For this review, take the finished solid that the model builds, in its own axes (mm). A direction names the side the tool comes from. Coordinates: 2 decimals unless noted, no trailing zeros. Write each loop counter-clockwise with the first axis right and the second up, starting at its lowest first coordinate (ties: lowest second). Pieces come first, ordered by that corner, then holes.
1) Insertion check: P1, Ø3, axis at x = 1.5, z = 10.5, coming from the -Y side; P2, Ø1.2, axis at y = 0, z = 13.5, coming from the +X side; P3, Ø1, axis at x = 1.5, z = 12.5, coming from the +Y side; P4, Ø1.6, axis at x = 0, y = 0, coming from the -Z side. Each pin has a flat end and moves straight along its axis. Give the tip position at first contact, or say it passes through.
2) Mouldability with a two-part tool opening along X and no side actions: class faces 4 (the face through (-3.45, 0, 8)), 5 (the face through (-1.3, 1.3, 0)), 6 (the face through (0, 0, 9)) as pulls with the +X half, pulls with the -X half, needs draft (parallel to the pull), parting line crosses it, or undercut.
3) We need section B-B on z = 6.25. Write out the cut boundary in (x, y).
4) We need section C-C on z = 13.5. Write out the cut boundary in (x, y), then the cut area to 3 significant figures.
5) To check wall thickness, follow line 1 along Z through (x, y) = (0.95, 0); line 2 along Z through (x, y) = (-1, -2.75); line 3 along Y through (x, z) = (0, 3.5). State the ranges of each line that lie inside material, in increasing order.
6) For faces 1 (the face through (1.7, 3, 7.7)), 2 (the face through (-0.17, -1.29, 4.7)), 3 (the face through (-2, -2, 10)), list the 3-axis set-ups (+Z, -Z, +X, -X, +Y, -Y) from which the entire face can be reached by the end or side of a thin tool; tool diameter is ignored.
from build123d import *

# Parameters (mm, degrees)
F2_R          = 5.941705
F3_DEPTH      = 16.501
F4_R          = 0.75
F5_DEPTH      = 3.451
F5_DEPTH_BACK = 3.451
F6_SIZE       = 0.3
F7_SIZE2      = 0.519615
F7_SIZE       = 0.3


with BuildPart() as f1:
    # F0 (on Front) → F1 (revolve)
    with BuildSketch(Plane.XZ):
        with BuildLine():
            Line((1.3, 9), (1.3, 0))
            Line((1.3, 0), (3.4, 0))
            Line((3.4, 0), (3.4, 5.5))
            Line((3.4, 5.5), (4, 5.66077))
            Line((4, 5.66077), (4, 9.83923))
            Line((4, 9.83923), (3.4, 10))
            Line((3.4, 10), (2.5, 10))
            ThreePointArc((2.5, 10), (2.146447, 10.146447), (2, 10.5))
            Line((2, 10.5), (2, 16))
            ThreePointArc((2, 16), (1.853553, 16.353553), (1.5, 16.5))
            Line((1.5, 16.5), (0, 16.5))
            Line((0, 16.5), (0, 9))
            Line((0, 9), (1.3, 9))
        make_face()
    revolve(axis=Axis((0, 0, 7.769906), (0, 0, -1)))

    # F2 (on Top) → F3 (cut, through all)
    with BuildSketch(Plane.XY):
        with Locations((0, -0.622483)):
            Circle(F2_R)
        Polygon((0, 3.983717), (3.45, 1.991858), (3.45, -1.991858), (0, -3.983717), (-3.45, -1.991858), (-3.45, 1.991858), align=None, mode=Mode.SUBTRACT)
    extrude(amount=F3_DEPTH, mode=Mode.SUBTRACT)

    # F4 (on Right) → F5 (cut, two sides)
    with BuildSketch(Plane.YZ) as f5_sk:
        with Locations((0, 13.5)):
            Circle(F4_R)
    extrude(amount=F5_DEPTH, mode=Mode.SUBTRACT)
    extrude(f5_sk.sketch, amount=-F5_DEPTH_BACK, mode=Mode.SUBTRACT)

    # F6
    f6_edges = [f1.edges().sort_by_distance(p)[0] for p in [
        (-3.4, 0, 0),
    ]]
    chamfer(f6_edges, length=F6_SIZE)

    # F7
    f7_edges = [f1.edges().sort_by_distance(p)[0] for p in [
        (-1.3, 0, 0),
    ]]
    chamfer(f7_edges, length=F7_SIZE, length2=F7_SIZE2)


solid = f1.part
Result:
1. P1: stops at y = -3.9
1. P2: passes through
1. P3: stops at y = 1.73
1. P4: stops at z = 9
2. face 4: pulls with the -X half
2. face 5: needs draft
2. face 6: undercut
3. outline: (-3.45, -1.99) - (0, -3.98) - (3.45, -1.99) - (3.45, 1.99) - (0, 3.98) - (-3.45, 1.99) - close; hole circle Ø2.6 at (0, 0)
4. outline: (-1.85, -0.75) arc R2 ccw to (1.85, -0.75) - close; (-1.85, 0.75) - (1.85, 0.75) arc R2 ccw to start
4. area: 6.71 mm2
5. line 1: z = 9 to 12.75, 14.25 to 16.5
5. line 2: z = 0 to 10
5. line 3: y = -3.4 to -1.3, 1.3 to 3.4
6. face 1: +Z, -Z, +X, +Y
6. face 2: -Z
6. face 3: +Z
